For this review, take the finished solid that the model builds, in its own axes (mm). A direction names the side the tool comes from. Round coordinates to 2 decimals unless told otherwise and drop trailing zeros. Write each loop counter-clockwise with the first axis right and the second up, starting at its lowest first coordinate (ties: lowest second). Pieces come first, ordered by that corner, then holes. Notation, with made-up numbers: M -0.5,-25.75 L 53.5,-25.75 A27 ccw 53.5,6.25 Z; hole C 53.25,4 d11. An arc over 180 degrees is marked long. Answer in a Markdown table with one row per item.
```python
from build123d import *

# Parameters (mm, degrees)
BOSS_EXTRUDE1_DEPTH = 25.4
SKETCH2_R           = 6.35
CUT_EXTRUDE1_DEPTH  = 169.886126132
FILLET1_R           = 19.05


with BuildPart() as part:
    # Sketch1 → Boss-Extrude1 (new body)
    with BuildSketch(Plane(origin=(0, 0, 0), x_dir=(1, 0, 0), z_dir=(0, 1, 0))):
        Polygon((-127, 6.35), (127, 6.35), (127, 85.09), (139.7, 85.09), (139.7, -6.35), (127, -6.35), (-127, -6.35), (-139.7, -6.35), (-139.7, 85.09), (-127, 85.09), align=None)
    extrude(amount=BOSS_EXTRUDE1_DEPTH)

    # Sketch2 → Cut-Extrude1 (cut, through all)
    with BuildSketch(Plane.XY.offset(6.35)):
        with Locations((0, 12.7)):
            Circle(SKETCH2_R)
    extrude(amount=-CUT_EXTRUDE1_DEPTH, mode=Mode.SUBTRACT)

    # Fillet1
    fillet1_edges = [part.edges().sort_by_distance(p)[0] for p in [
        (-139.7, 12.7, 6.35),
        (-127, 12.7, -6.35),
        (127, 12.7, -6.35),
        (139.7, 12.7, 6.35),
    ]]
    fillet(fillet1_edges, radius=FILLET1_R)


solid = part.part
```
Q1. Take a section at B-B (x = 0). State the section outline as (y, z) points, then the cut area to 3 significant figures.
Found:
| item | result |
|---|---|
| outline | M 0,-6.35 L 6.35,-6.35 L 6.35,6.35 L 0,6.35 Z; M 19.05,-6.35 L 25.4,-6.35 L 25.4,6.35 L 19.05,6.35 Z |
| area | 161 mm² |
Q2. Machinability: for faces 4 (the face through (121.27, 12.88, -11.78)), 5 (the face through (133, 13, -85.09)), which of the approach directions +Z, -Z, +X, -X, +Y, -Y give a long, thin tool a straight path to every point of the face, cutting with its end or side? Answer none if there is none.
Found:
| item | result |
|---|---|
| face 4 | -Z, +Y, -Y |
| face 5 | -Z, +X, -X, +Y, -Y |
Q3. Take a section at C-C (z = -40). State the section outline as (x, y) points, then the cut area to 3 significant figures.
Found:
| item | result |
|---|---|
| outline | M -139.7,0 L -127,0 L -127,25.4 L -139.7,25.4 Z; M 127,0 L 139.7,0 L 139.7,25.4 L 127,25.4 Z |
| area | 645 mm² |
Q4. Insertion check: P1, Ø4, axis at x = -4, y = 4.5, coming from the -Z side. The pin has a flat end and moves straight along its axis. Give the tip position at first contact, or say it passes through.
Found:
| item | result |
|---|---|
| P1 | z = -6.35 |
Q5. Take a section at D-D (x = 50.5). State the section outline as (y, z) points.
Found:
| item | result |
|---|---|
| outline | M 0,-6.35 L 25.4,-6.35 L 25.4,6.35 L 0,6.35 Z |
Q6. Take a section at A-A (y = 12.7). State the section outline as (x, z) points, then the cut area to 3 significant figures.
Found:
| item | result |
|---|---|
| outline | M -139.7,-85.09 L -127,-85.09 L -127,-25.4 A19.05 cw -107.95,-6.35 L -6.35,-6.35 L -6.35,6.35 L -120.65,6.35 A19.05 ccw -139.7,-12.7 Z; M 6.35,-6.35 L 107.95,-6.35 A19.05 cw 127,-25.4 L 127,-85.09 L 139.7,-85.09 L 139.7,-12.7 A19.05 ccw 120.65,6.35 L 6.35,6.35 Z |
| area | 5,390 mm² |
Q7. Mouldability with a two-part tool opening along Y and no side actions: class faces 1 (the face through (-127, 13, -56)), 2 (the face through (3.414, 18.054, 0.089)), 3 (the face through (1, 25.4, -6)) as +Y half, -Y half, draft (parallel to the pull), parting line (faces both ways), or undercut.
Found:
| item | result |
|---|---|
| face 1 | draft |
| face 2 | undercut |
| face 3 | +Y half |
Q8. For probe 1 along X at (y, z) = (3.5, -71); probe 2 along Y at (x, z) = (0, -0.25); probe 3 along Z at (x, y) = (-109, 11.75), list the stretches that pass through material, from the lowest coordinate up.
Found:
| item | result |
|---|---|
| probe 1 | -139.7 to -127, 127 to 139.7 |
| probe 2 | 0 to 6.35, 19.05 to 25.4 |
| probe 3 | -6.38 to 6.35 |
